Autodesk Inventor part; units mm, degrees
ref_plane "YZ Plane" through (0, 0, 0) normal (1, 0, 0) x (0, 1, 0)
ref_plane "XZ Plane" through (0, 0, 0) normal (0, 1, 0) x (-1, 0, 0)
ref_plane "XY Plane" through (0, 0, 0) normal (0, 0, 1) x (1, 0, 0)
sketch "Sketch1" plane through (0, 0, 0) normal (0, 1, 0) x (-1, 0, 0)
  circle A0 centre (42.5, 0) radius 2
  circle A1 centre (-21.25, 36.8061) radius 2
  circle A2 centre (-21.25, -36.8061) radius 2
  line L0 (-21.25, -36.8061) -> (0, 0) construction
  arc A3 (-25.1562, -34.5508) -> (-20.8492, -41.2987) centre (-21.25, -36.8061) ccw
  line L1 (-21.25, 36.8061) -> (0, 0) construction
  arc A4 (-17.3438, 39.0613) -> (-25.1562, 34.5508) centre (-21.25, 36.8061) ccw
  line L2 (0, 0) -> (42.5, 0) construction
  arc A5 (42.5, -4.5105) -> (42.5, 4.5105) centre (42.5, 0) ccw
  line L3 (-21.6508, -41.2987) -> (28.2014, -41.2987)
  line L4 (28.2014, -41.2987) -> (33.3458, -35.9407)
  line L5 (33.3458, -35.9407) -> (33.3458, -15.3261)
  line L6 (-25.1562, -34.5508) -> (-22.1167, -29.2863)
  line L7 (36.421, -4.5105) -> (42.5, -4.5105)
  line L8 (42.5, 0) -> (36.6992, 0)
  line L9 (4.5105, 0) -> (0, 0)
  line L10 (42.5, 4.5105) -> (36.421, 4.5105)
  line L11 (-25.1562, 34.5508) -> (-22.1167, 29.2863)
  line L12 (-14.3043, 33.7968) -> (-17.3438, 39.0613)
  arc A6 (-22.1167, 29.2863) -> (-22.1167, -29.2863) centre (0, 0) ccw
  arc A7 (33.3458, -15.3261) -> (36.421, -4.5105) centre (0, 0) ccw
  arc A8 (36.421, 4.5105) -> (-14.3043, 33.7968) centre (0, 0) ccw
  point P0 (-10.625, -18.403)
  point P1 (-10.625, 18.403)
  point P2 (21.25, 0)
  dimension "d1" = 4
  dimension "d2" = 42.5
  dimension "d5" = 360
extrude "Extrusion1" add sketch "Sketch1" along normal blind 1.6 contours L6 A6 L11 A4 L12 A8 L10 A5 L7 A7 L5 L4 L3 A3
sketch "Sketch2" plane through (0, 1.6, 0) normal (0, 1, 0) x (1, 0, 0)
  line L0 (35, 0) -> (0, 0) construction
  circle A0 centre (12.5, 12.5) radius 3
  circle A1 centre (-12.5, 12.5) radius 3
  circle A2 centre (-12.5, -12.5) radius 3
  circle A3 centre (12.5, -12.5) radius 3
  line L1 (1.675, -1.675) -> (-1.675, -1.675)
  line L2 (-1.675, -1.675) -> (-1.675, 1.675)
  line L3 (-1.675, 1.675) -> (1.675, 1.675)
  line L4 (1.675, 1.675) -> (1.675, -1.675)
  line L5 (1.675, -1.675) -> (-1.675, 1.675) construction
  line L6 (-1.675, -1.675) -> (1.675, 1.675) construction
  circle A4 centre (0, 0) radius 1.675
  circle A5 centre (0, -28) radius 3.75
  line L7 (0, -28) -> (0, 0) construction
  line L8 (-42.5, -4.5105) -> (-36.421, -4.5105)
  arc A6 (-42.5, 4.5105) -> (-42.5, -4.5105) centre (-42.5, 0) ccw
  line L9 (-36.421, 4.5105) -> (-42.5, 4.5105)
  arc A7 (-33.3458, 15.3261) -> (-36.421, 4.5105) centre (0, 0) ccw
  line L10 (-33.3458, 35.9407) -> (-33.3458, 15.3261)
  line L11 (-28.2014, 41.2987) -> (-33.3458, 35.9407)
  line L12 (21.6508, 41.2987) -> (-28.2014, 41.2987)
  arc A8 (25.1562, 34.5508) -> (21.6508, 41.2987) centre (21.25, 36.8061) ccw
  line L13 (22.1167, 29.2863) -> (25.1562, 34.5508)
  arc A9 (22.1167, -29.2863) -> (22.1167, 29.2863) centre (0, 0) ccw
  line L14 (25.1562, -34.5508) -> (22.1167, -29.2863)
  arc A10 (17.3438, -39.0613) -> (25.1562, -34.5508) centre (21.25, -36.8061) ccw
  line L15 (14.3043, -33.7968) -> (17.3438, -39.0613)
  arc A11 (-36.421, -4.5105) -> (14.3043, -33.7968) centre (0, 0) ccw
  circle A12 centre (21.25, 36.8061) radius 2
  circle A13 centre (21.25, -36.8061) radius 2
  circle A14 centre (-42.5, 0) radius 2
  circle A15 centre (11, 38.1) radius 0.381
  circle A16 centre (14.4, 38.1) radius 0.381
  line L16 (11, 38.1) -> (14.4, 38.1) construction
  dimension "d23" = 35
  dimension "d24" = 360
  dimension "d25" = 12.5
  dimension "d26" = 12.5
  dimension "d27" = 6
  dimension "d28" = 360
  dimension "d31" = 3.35
  dimension "d32" = 28
  dimension "d33" = 7.5
  dimension "d34" = 11
  dimension "d36" = 38.1
  dimension "d37" = 3.4
  dimension "d38" = 0.762
extrude "Extrusion2" cut sketch "Sketch2" against normal blind 0.5 contours A0 | A1 | A2 | A3 | A4 | A5 | A15 | A16
sketch "Sketch3" plane through (0, 0, 0) normal (0, -1, 0) x (1, 0, 0)
  line L0 (14.38, -37.6973) -> (11.88, -37.6973)
  line L1 (21.6508, -41.2987) -> (-28.2014, -41.2987) construction
  line L2 (11.88, -32.9109) -> (14.38, -32.9109)
  arc A0 (14.38, -37.6973) -> (14.38, -32.9109) centre (13.13, -35.3041) ccw
  arc A1 (11.88, -32.9109) -> (11.88, -37.6973) centre (13.13, -35.3041) ccw
  line L3 (11.88, -37.6973) -> (14.38, -32.9109) construction
  line L4 (14.38, -37.6973) -> (11.88, -32.9109) construction
  line L5 (14.4, -35.3041) -> (11.86, -35.3041) construction
  circle A2 centre (14.4, -35.3041) radius 0.381
  circle A3 centre (11.86, -35.3041) radius 0.381
  circle A4 centre (21.25, -36.8061) radius 2 construction
  point P0 (0, 0)
  dimension "d39" = 2.7
  dimension "d40" = 2.5
  dimension "d41" = 0.762
  dimension "d42" = 2.54
  dimension "d43" = 6.85
  dimension "d44" = 1.502
extrude "Extrusion3" add sketch "Sketch3" along normal blind 1 contours L0 A1 L2 A0 | A2 | A3
properties part number "PCB"
Design review of the part built by this model. Coordinates are the model's own, in mm. A direction names the side the tool comes from. Coordinates: 2 decimals unless noted, no trailing zeros. Order: outer loops, then holes, each group sorted by start corner. A loop starts at its lowest first (then second) coordinate and runs counter-clockwise, first axis right, second up.
Item 1: The part is to be moulded in two halves that separate along X. For faces 6 (the flat face through (-30.738, 0.789, -38.657)), 7 (the cylindrical face through (25.223, 0.789, -38.941)), 8 (the cylindrical face through (-14.9, 1.4, -10.7)), say which applies: pulls with the +X half, pulls with the -X half, needs draft (parallel to the pull), parting line crosses it, or undercut.
Item 2: Take a section at B-B, the plane x = -12. Write out the cut boundary in (y, z), then the cut area to 3 significant figures.
Item 3: Take a section at C-C, the plane y = 0.65. Write out the cut boundary in (x, z).
Item 4: Take a section at A-A, the plane z = 0. Write out the cut boundary in (x, y) (1 decimal), then the cut area to 3 significant figures.
Item 5: For pin 1 Ø0.5 at (x, y) = (12.5, -0.5) entering from +Z; pin 2 Ø5 at (x, z) = (-0.5, 11) entering from -Y; pin 3 Ø1.8 at (x, z) = (-13, -12.5) entering from +Y, all flat-tipped, find the tip position at first contact; note any pin that passes through.
Item 6: For faces 1 (the flat face through (-5, 1.6, 1)), 2 (the flat face through (23.66, 0.79, -31.96)), 3 (the flat face through (-13, 1.1, -13)), 4 (the cylindrical face through (-47.01, 0.79, 0.1)), 5 (the flat face through (15.8, 0.79, 36.39)), list the 3-axis set-ups (+Z, -Z, +X, -X, +Y, -Y) from which the entire face can be reached by the end or side of a thin tool; tool diameter is ignored.
Item 7: Take a section at D-D, the plane z = 12.5. Write out the cut boundary in (x, y).
Item 8: For line 1 (Z direction, x = 0, y = 1.35) (3 decimals); line 2 (X direction, y = 1.3, z = -12.5); line 3 (Z direction, x = 11, y = 1.25), list the stretches that pass through material, from the lowest coordinate up.
The answers:
1. face 6: pulls with the -X half
1. face 7: pulls with the +X half
1. face 8: undercut
2. outline: (0, -41.3) - (1.6, -41.3) - (1.6, -15.46) - (1.1, -15.46) - (1.1, -9.54) - (1.6, -9.54) - (1.6, 9.54) - (1.1, 9.54) - (1.1, 15.46) - (1.6, 15.46) - (1.6, 34.68) - (0, 34.68) - close
2. area: 116 mm2
3. outline: (-42.5, -4.51) - (-36.42, -4.51) arc R36.7 ccw to (-33.35, -15.33) - (-33.35, -35.94) - (-28.2, -41.3) - (21.65, -41.3) arc R4.51 ccw to (25.16, -34.55) - (22.12, -29.29) arc R36.7 ccw to (22.12, 29.29) - (25.16, 34.55) arc R4.51 ccw to (17.34, 39.06) - (14.3, 33.8) arc R36.7 ccw to (-36.42, 4.51) - (-42.5, 4.51) arc R4.51 ccw to start; hole circle Ø4 at (-42.5, 0); hole circle Ø4 at (21.25, -36.81); hole circle Ø4 at (21.25, 36.81)
4. outline: (-47, 0) - (-44.5, 0) - (-44.5, 1.6) - (-47, 1.6) - close; (-40.5, 0) - (36.7, 0) - (36.7, 1.6) - (1.7, 1.6) - (1.7, 1.1) - (-1.7, 1.1) - (-1.7, 1.6) - (-40.5, 1.6) - close
4. area: 126 mm2
5. pin 1: stops at z = -32.91
5. pin 2: stops at y = 0
5. pin 3: stops at y = 1.1
6. face 1: +Z, -Z, +X, -X, +Y
6. face 2: +X, +Y, -Y
6. face 3: +Y
6. face 4: -X, +Y, -Y
6. face 5: +Z, +Y, -Y
7. outline: (-34.5, 0) - (34.5, 0) - (34.5, 1.6) - (15.5, 1.6) - (15.5, 1.1) - (9.5, 1.1) - (9.5, 1.6) - (-9.5, 1.6) - (-9.5, 1.1) - (-15.5, 1.1) - (-15.5, 1.6) - (-34.5, 1.6) - close
8. line 1: z = -41.299 to -1.675, 1.675 to 24.25, 31.75 to 36.699
8. line 2: x = -34.5 to -15.5, -9.5 to 9.5, 15.5 to 34.5
8. line 3: z = -41.3 to -38.48, -37.72 to -15.1, -9.9 to 9.9, 15.1 to 35.01
